Check sheet for the drawn part. Datum: minimum x, y, z corner. Units: mm. A direction names the side the tool comes from. Coordinates: 2 decimals unless noted, no trailing zeros. Write each loop counter-clockwise with the first axis right and the second up, starting at its lowest first coordinate (ties: lowest second). Pieces come first, ordered by that corner, then holes. Notation, with made-up numbers: M -19,-10.5 L 14,-10.5 A19 cw 14,16.5 Z; hole C 89.25,30 d10. An arc over 180 degrees is marked long. Answer in a Markdown table with one row per item.
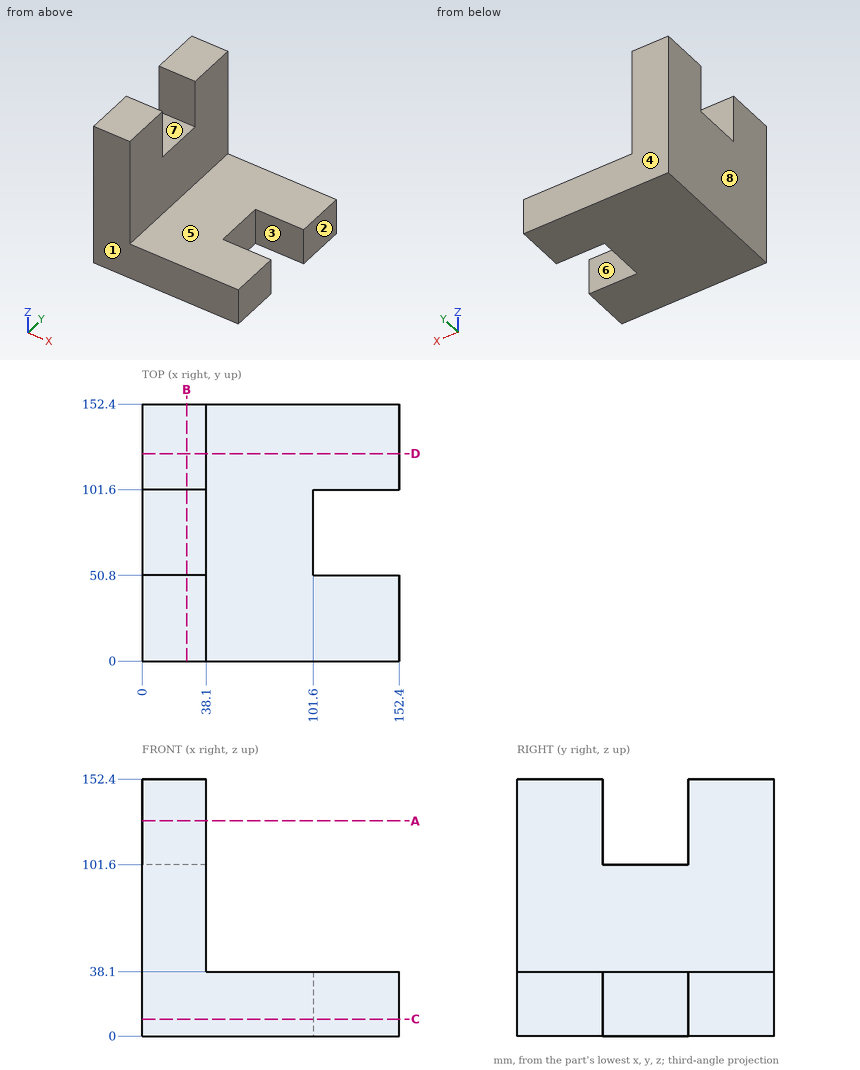
1) Sectioned sample at A-A (z = 127.5). Record the cut outline in (x, y), then the cut area to 3 significant figures.
Response values:
| item | result |
|---|---|
| outline | M 0,0 L 38.1,0 L 38.1,50.8 L 0,50.8 Z; M 0,101.6 L 38.1,101.6 L 38.1,152.4 L 0,152.4 Z |
| area | 3,870 mm² |
2) Sectioned sample at D-D (y = 123). Record the cut outline in (x, z).
Response values:
| item | result |
|---|---|
| outline | M 0,0 L 152.4,0 L 152.4,38.1 L 38.1,38.1 L 38.1,152.4 L 0,152.4 Z |
3) Tool access check on the marked faces 5, 6, 7 and 8. Record the directions out of +Z, -Z, +X, -X, +Y, -Y that give a thin tool (end or side, any length) a straight path to the whole face; none if there is none.
Response values:
| item | result |
|---|---|
| face 5 | +Z, +X, +Y, -Y |
| face 6 | +Z, -Z, +X |
| face 7 | +Z, +X, -X |
| face 8 | +Z, -Z, -X, +Y, -Y |
4) Sectioned sample at B-B (x = 26.5). Record the cut outline in (y, z).
Response values:
| item | result |
|---|---|
| outline | M 0,0 L 152.4,0 L 152.4,152.4 L 101.6,152.4 L 101.6,101.6 L 50.8,101.6 L 50.8,152.4 L 0,152.4 Z |
5) Sectioned sample at C-C (z = 10). Record the cut outline in (x, y), then the cut area to 3 significant figures.
Response values:
| item | result |
|---|---|
| outline | M 0,0 L 152.4,0 L 152.4,50.8 L 101.6,50.8 L 101.6,101.6 L 152.4,101.6 L 152.4,152.4 L 0,152.4 Z |
| area | 20,600 mm² |
6) Thickness scan on L1, parallel to Y at x = 30.5, z = 129.5; L2, parallel to X at y = 46, z = 141. Record the ranges inside material, lowest first. Write a range as [from, to].
Response values:
| item | result |
|---|---|
| L1 | y = [0, 50.8], [101.6, 152.4] |
| L2 | x = [0, 38.1] |
7) Depth check by flat-ended pin: pin 1 (19 mm diameter, centred on y = 88, z = 20.5, fed in from +X); pin 2 (1.5 mm diameter, centred on x = 116, y = 118, fed in from +Z); pin 3 (1 mm diameter, centred on x = 21, y = 82, fed in from +Z). Enter the tip coordinate at first touch or a pass-through.
Response values:
| item | result |
|---|---|
| pin 1 | stops at x = 101.6 |
| pin 2 | stops at z = 38.1 |
| pin 3 | stops at z = 101.6 |
8) Release check for a two-part mould opening along Y. For the marked faces 1, 2, 3 and 4 record: +Y half, -Y half, draft (parallel to the pull), parting line (faces both ways), or undercut.
Response values:
| item | result |
|---|---|
| face 1 | -Y half |
| face 2 | draft |
| face 3 | undercut |
| face 4 | +Y half |
